Can you work these out from the model? Positions are in its coordinate system, mm. Coordinates: 2 decimals unless noted, no trailing zeros. Order: outer loops, then holes, each group sorted by start corner. A loop starts at its lowest first (then second) coordinate and runs counter-clockwise, first axis right, second up. Notation, with made-up numbers: M 28.5,-15.5 L 74.5,-15.5 A17 cw 74.5,-9.5 Z; hole C -12.5,63 d3. An arc over 180 degrees is marked long. Answer as CSV lines item,"result". Start each with the question number.
1. If we section it at B-B (z = 764): List the corners of the cut face in (x, y) for me.
2. If we section it at A-A (x = 11.5): List the corners of the cut face in (y, z) for me, plus the area to 3 significant figures.
3. Will these pins go through, and if not, where does the flat tip stop? pin 1 (3 mm diameter, centred on x = -26, z = 150, fed in from -Y); pin 2 (2 mm diameter, centred on y = -18, z = 662, fed in from +X).
4. I need wall thicknesses on line 1 along X through (y, z) = (-27, 955); line 2 along Z through (x, y) = (23, -26.8); line 3 along Y through (x, z) = (-29.65, 175). Which ranges of each line are inside material? Lowest first, please. Write a range as from..to.
5. If we section it at C-C (y = 8): List the corners of the cut face in (x, z) for me, plus the area to 3 significant figures.
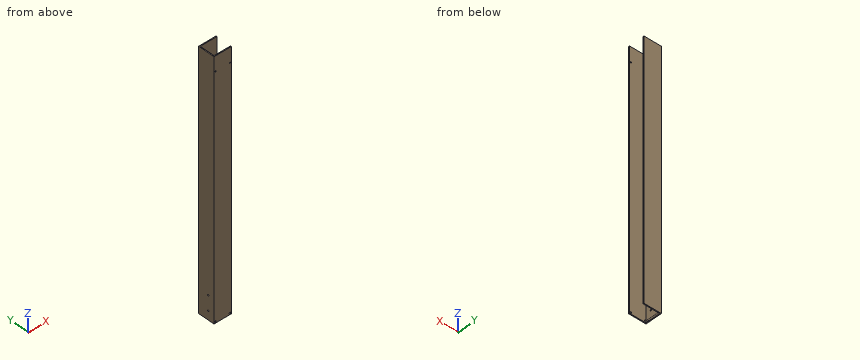
```python
from build123d import *

# Parameters (mm, degrees)
ESTRUSIONE_ESTRUSIONE1_DEPTH = 1005
SCHIZZO2_R                   = 2
TAGLIO_ESTRUSIONE1_DEPTH     = 50
SCHIZZO3_R                   = 2.5
TAGLIO_ESTRUSIONE2_DEPTH     = 50
SCHIZZO4_W                   = 59
SCHIZZO4_H                   = 145
TAGLIO_ESTRUSIONE3_DEPTH     = 63
SCHIZZO8_R                   = 2.5
TAGLIO_ESTRUSIONE5_DEPTH     = 10


with BuildPart() as part:
    # Schizzo1 → Estrusione-Estrusione1 (new body)
    with BuildSketch(Plane.XY):
        Polygon((28, -25), (28, -28), (-31, -28), (-31, 28), (28, 28), (28, 25), (-28, 25), (-28, -25), align=None)
    extrude(amount=ESTRUSIONE_ESTRUSIONE1_DEPTH)

    # Schizzo2 → Taglio-Estrusione1 (cut)
    with BuildSketch(Plane(origin=(0, -28, 0), x_dir=(-1, 0, 0), z_dir=(0, -1, 0))):
        with Locations((-23, -955)):
            Circle(SCHIZZO2_R)
        with Locations((26, -955)):
            Circle(SCHIZZO2_R)
    extrude(amount=-TAGLIO_ESTRUSIONE1_DEPTH, mode=Mode.SUBTRACT)

    # Schizzo3 → Taglio-Estrusione2 (cut)
    with BuildSketch(Plane(origin=(0, -28, 0), x_dir=(-1, 0, 0), z_dir=(0, -1, 0))):
        with Locations((26, -150)):
            Circle(SCHIZZO3_R)
        with Locations((-23, -150)):
            Circle(SCHIZZO3_R)
    extrude(amount=-TAGLIO_ESTRUSIONE2_DEPTH, mode=Mode.SUBTRACT)

    # Schizzo4 → Taglio-Estrusione3 (cut)
    with BuildSketch(Plane(origin=(0, 28, 0), x_dir=(1, 0, 0), z_dir=(0, 1, 0))):
        with Locations((-1.5, -72.5)):
            Rectangle(SCHIZZO4_W, SCHIZZO4_H)
    extrude(amount=-TAGLIO_ESTRUSIONE3_DEPTH, mode=Mode.SUBTRACT)

    # Schizzo8 → Taglio-Estrusione5 (cut)
    with BuildSketch(Plane.ZY.offset(31)):
        with Locations((175, -7)):
            Circle(SCHIZZO8_R)
        with Locations((225, -7)):
            Circle(SCHIZZO8_R)
    extrude(amount=-TAGLIO_ESTRUSIONE5_DEPTH, mode=Mode.SUBTRACT)


solid = part.part
```
Solved:
1,outline,"M -31,-28 L 28,-28 L 28,-25 L -28,-25 L -28,25 L 28,25 L 28,28 L -31,28 Z"
2,outline,"M -28,145 L -25,145 L -25,1005 L -28,1005 Z; M 25,145 L 28,145 L 28,1005 L 25,1005 Z"
2,area,"5,160 mm²"
3,pin 1,"y = 25"
3,pin 2,"x = -28"
4,line 1,"-31..-28, -24..21, 25..28"
4,line 2,"145..147.5, 152.5..953, 957..1005"
4,line 3,"-28..-9.5, -4.5..28"
5,outline,"M -31,145 L -28,145 L -28,148.5 A2.5 cw -28,151.5 L -28,1005 L -31,1005 Z"
5,area,"2,580 mm²"
